Verification items for the finished model (mm, model axes). A direction names the side the tool comes from. Round coordinates to 2 decimals unless told otherwise and drop trailing zeros. Order: outer loops, then holes, each group sorted by start corner. A loop starts at its lowest first (then second) coordinate and runs counter-clockwise, first axis right, second up. Notation, with made-up numbers: M -26,43 L 33,43 A38 ccw 33,82 Z; hole C -36.5,27.5 d9. An arc over 180 degrees is marked long. Answer as a JSON object with one key per item and string values. Group by question number.
```python
from build123d import *

# Parameters (mm, degrees)
SKETCH_4_R          = 2.5
EXTRUDE_1_DEPTH     = 5
SKETCH_5_W          = 5
SKETCH_5_H          = 5
CUT_EXTRUDE_5_DEPTH = 5
FILLET_1_R          = 5


with BuildPart() as part:
    # 草图4 → 凸台-拉伸1 (new body)
    with BuildSketch(Plane.XY):
        Polygon((-30.514243596, -31.085830111), (29.485756404, -31.085830111), (29.485756404, 33.914169889), (-30.514243596, 33.914169889), (-45.514243596, 33.914169889), (-45.514243596, -31.085830111), align=None)
        with Locations((23.135756404, 24.289169889)):
            Circle(SKETCH_4_R, mode=Mode.SUBTRACT)
        with Locations((23.135756404, 14.289169889)):
            Circle(SKETCH_4_R, mode=Mode.SUBTRACT)
        with Locations((23.135756404, -11.050830111)):
            Circle(SKETCH_4_R, mode=Mode.SUBTRACT)
        with Locations((23.135756404, -21.050830111)):
            Circle(SKETCH_4_R, mode=Mode.SUBTRACT)
        with Locations((-26.364243596, -21.050830111)):
            Circle(SKETCH_4_R, mode=Mode.SUBTRACT)
        with Locations((-26.364243596, -11.050830111)):
            Circle(SKETCH_4_R, mode=Mode.SUBTRACT)
        with Locations((-26.364243596, 14.289169889)):
            Circle(SKETCH_4_R, mode=Mode.SUBTRACT)
        with Locations((-26.364243596, 24.289169889)):
            Circle(SKETCH_4_R, mode=Mode.SUBTRACT)
        Polygon((-27.614243596, -17.050830111), (-21.614243596, -17.050830111), (-21.614243596, -26.550830111), (18.485756404, -26.550830111), (18.485756404, -17.050830111), (25.485756404, -17.050830111), (25.485756404, -15.050830111), (18.485756404, -15.050830111), (18.485756404, -5.550830111), (-21.614243596, -5.550830111), (-21.614243596, -15.050830111), (-27.614243596, -15.050830111), align=None, mode=Mode.SUBTRACT)
        Polygon((18.485756404, 29.789169889), (-21.614243596, 29.789169889), (-21.614243596, 20.289169889), (-27.614243596, 20.289169889), (-27.614243596, 18.289169889), (-21.614243596, 18.289169889), (-21.614243596, 8.789169889), (18.485756404, 8.789169889), (18.485756404, 18.289169889), (25.485756404, 18.289169889), (25.485756404, 20.289169889), (18.485756404, 20.289169889), align=None, mode=Mode.SUBTRACT)
    extrude(amount=EXTRUDE_1_DEPTH)

    # 草图5 → 切除-拉伸5 (cut)
    with BuildSketch(Plane(origin=(0, 0, 0), x_dir=(-1, 0, 0), z_dir=(0, 0, -1))):
        Polygon((40.514243596, -1.085830111), (40.514243596, 1.414169889), (40.514243596, 3.914169889), (35.514243596, 3.914169889), (35.514243596, -1.085830111), align=None)
        with Locations((38.014243596, 19.414169889)):
            Rectangle(SKETCH_5_W, SKETCH_5_H)
        with Locations((38.014243596, -16.585830111)):
            Rectangle(SKETCH_5_W, SKETCH_5_H)
    extrude(amount=-CUT_EXTRUDE_5_DEPTH, mode=Mode.SUBTRACT)

    # 圆角1
    fillet_1_edges = [part.edges().sort_by_distance(p)[0] for p in [
        (-45.514243596, -31.085830111, 2.5),
        (-45.514243596, 33.914169889, 2.5),
        (29.485756404, 33.914169889, 2.5),
        (29.485756404, -31.085830111, 2.5),
    ]]
    fillet(fillet_1_edges, radius=FILLET_1_R)


solid = part.part
```
Q1. Release check for a two-part mould opening along X. For faces 1 (the face through (28.06, 32.41, 2.54)), 2 (the face through (-45.514, 2, 2)), 3 (the face through (22, -15.051, 2)) record: released by +X, released by -X, zero draft, split by the parting line, or undercut.
Q2. Thickness scan on line 1 (X direction, y = 24.5, z = 1); line 2 (Y direction, x = 0, z = 2.45); line 3 (X direction, y = -16, z = 3.3). Record the ranges inside material, lowest first. Write a range as from..to.
Q3. Cross-section at A-A, the plane y = -25. Record the cut outline in (x, z).
Q4. Cross-section at B-B, the plane x = -13. Record the cut outline in (y, z).
Q5. Cross-section at C-C, the plane z = 3.2. Give the number of separate pieces and of enclosed holes in the cut face, then the cut area to 3 significant figures.
Q6. Tool access check on faces 4 (the face through (-40.514, 1, 2)), 5 (the face through (-17, 2, 0)). Record the directions out of +Z, -Z, +X, -X, +Y, -Y that give a thin tool (end or side, any length) a straight path to the whole face; none if there is none.
Conclusion:
{
 "1": {"face 1": "released by +X", "face 2": "released by -X", "face 3": "undercut"},
 "2": {"line 1": "-45.51..-28.86, -23.87..-21.61, 18.49..20.64, 25.63..29.49", "line 2": "-31.09..-26.55, -5.55..8.79, 29.79..33.91", "line 3": "-45.51..-40.51, -35.51..-27.61, 25.49..29.49"},
 "3": {"outline": "M -45.51,0 L -21.61,0 L -21.61,5 L -45.51,5 Z; M 18.49,0 L 29.49,0 L 29.49,5 L 18.49,5 Z"},
 "4": {"outline": "M -31.09,0 L -26.55,0 L -26.55,5 L -31.09,5 Z; M -5.55,0 L 8.79,0 L 8.79,5 L -5.55,5 Z; M 29.79,0 L 33.91,0 L 33.91,5 L 29.79,5 Z"},
 "5": {"separate pieces": "1", "enclosed holes": "13", "area": "2,890 mm2"},
 "6": {"face 4": "+Z, -Z", "face 5": "-Z, +X, -X, +Y, -Y"}
}
